```python
from build123d import *

# Parameters (mm, degrees)
F1_DEPTH = 3.175
F2_R     = 3.175
F3_DEPTH = 6.351


with BuildPart() as f1:
    # F0 (on Right) → F1 (new body, symmetric)
    with BuildSketch(Plane.YZ):
        with BuildLine():
            Line((0, -12.7), (0, 0))
            Line((0, 0), (0, 12.7))
            ThreePointArc((0, 12.7), (-17.960512, 5.260512), (-25.4, -12.7))
            Line((-25.4, -12.7), (0, -12.7))
        make_face()
        with BuildLine():
            Line((0, 12.7), (0, 0))
            Line((0, 0), (12.7, 0))
            ThreePointArc((12.7, 0), (8.980256, 8.980256), (0, 12.7))
        make_face()
        with BuildLine():
            Line((12.7, 0), (0, 0))
            Line((0, 0), (0, -12.7))
            ThreePointArc((0, -12.7), (8.980256, -8.980256), (12.7, 0))
        make_face()
    extrude(amount=F1_DEPTH, both=True)

    # F2 (on face) → F3 (cut, through all)
    with BuildSketch(Plane.YZ.offset(3.175)):
        with Locations((0, -5.715)):
            Circle(F2_R)
    extrude(amount=-F3_DEPTH, mode=Mode.SUBTRACT)


solid = f1.part
```
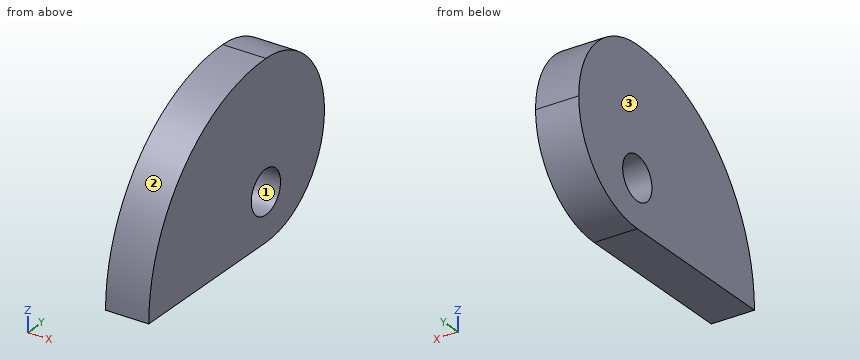
The listing builds one solid part. Answer for the finished solid, in the listing's coordinates (mm). Face numbers are marked on the shaded views. Coordinates: 2 decimals unless noted, no trailing zeros. Write each loop counter-clockwise with the first axis right and the second up, starting at its lowest first coordinate (ties: lowest second). Pieces come first, ordered by that corner, then holes. Notation, with made-up numbers: (-35, -0.5) - (-2, -0.5) arc R27 ccw to (-2, 18.5) - close; hole circle Ø9 at (57, 10.25). An arc over 180 degrees is marked (long way). Return JSON: item names as keys, results as strings. Group by question number.
1. A cutting plane is placed at D-D, the plane y = 2.5. Determine the outline of the cut face in (x, z) (1 decimal), plus the area to 3 significant figures.
2. A cutting plane is placed at A-A, the plane y = -1.5. Determine the outline of the cut face in (x, z) (3 decimals), plus the area to 3 significant figures.
3. Determine the mould class of the marked faces 1, 2 and 3 for opening direction Y: released by +Y, released by -Y, zero draft, split by the parting line, or undercut.
4. Given pin 1 (1 mm diameter, centred on x = -1.5, y = 8, fed in from -Z); pin 2 (1 mm diameter, centred on x = -2.5, z = 1, fed in from -Y); pin 3 (4 mm diameter, centred on y = 0, z = -5.715, fed in from -X); pin 4 (2 mm diameter, centred on x = 2, z = -0.5, fed in from +Y), each flat-ended and moving along its own axis, determine where each tip first touches the part or whether it passes through.
5. A cutting plane is placed at B-B, the plane x = 1.25. Determine the outline of the cut face in (y, z) (3 decimals).
6. A cutting plane is placed at C-C, the plane z = 4. Determine the outline of the cut face in (x, y) (3 decimals), plus the area to 3 significant figures.
7. Straight lines are drawn through the part: L1, parallel to Y at x = 2.25, z = -3.25; L2, parallel to Z at x = 0.25, y = -22; L3, parallel to Y at x = -2.5, z = 9.75. For each, find the intervals that lie inside material, in ascending order.
Ans:
{
 "1": {"outline": "(-3.2, -12.5) - (3.2, -12.5) - (3.2, -7.7) - (-3.2, -7.7) - close; (-3.2, -3.8) - (3.2, -3.8) - (3.2, 12.5) - (-3.2, 12.5) - close", "area": "133 mm²"},
 "2": {"outline": "(-3.175, -12.7) - (3.175, -12.7) - (3.175, -8.513) - (-3.175, -8.513) - close; (-3.175, -2.917) - (3.175, -2.917) - (3.175, 12.656) - (-3.175, 12.656) - close", "area": "125 mm²"},
 "3": {"face 1": "undercut", "face 2": "released by -Y", "face 3": "zero draft"},
 "4": {"pin 1": "z = -10.25", "pin 2": "y = -21.7", "pin 3": "through", "pin 4": "y = 12.7"},
 "5": {"outline": "(-25.4, -12.7) - (0, -12.7) arc R12.7 ccw to (0, 12.7) arc R25.4 ccw to start; hole circle Ø6.35 at (0, -5.715)"},
 "6": {"outline": "(-3.175, -19.138) - (3.175, -19.138) - (3.175, 12.054) - (-3.175, 12.054) - close", "area": "198 mm²"},
 "7": {"L1": "-23.58 to -2, 2 to 12.28", "L2": "-12.7 to -0.01", "L3": "-11.88 to 8.14"}
}
